```python
from build123d import *

# Parameters (mm, degrees)
BASE_FLANGE1_DEPTH         = 6
SKETCHED_START             = -292.5
SKETCHED_BEND1_OUTLINE_W   = 6
SKETCHED_BEND1_OUTLINE_H   = 180
SKETCHED_BEND1_DEPTH       = 75
SKETCHED_START_2           = 217.5
SKETCHED_BEND1_2_OUTLINE_W = 6
SKETCHED_BEND1_2_OUTLINE_H = 180
SKETCHED_BEND1_2_DEPTH     = 75
SKETCHED_START_3           = -217.5
SKETCHED_BEND1_3_DEPTH     = 6.7366
SKETCHED_START_4           = 210.7634
SKETCHED_BEND1_4_DEPTH     = 6.7366
SKETCHED_START_5           = -91
SKETCHED_BEND1_5_DEPTH     = 182


with BuildPart() as part:
    # Base-Flange1: sheet metal written as solids
    # Sketch1 → Base-Flange1 (new body)
    with BuildSketch(Plane(origin=(0, 0, 0), x_dir=(1, 0, 0), z_dir=(0, 1, 0))):
        with BuildLine():
            Line((-282.5, 90), (282.5, 90))
            ThreePointArc((282.5, 90), (289.571067812, 87.071067812), (292.5, 80))
            Line((292.5, 80), (292.5, -80))
            ThreePointArc((292.5, -80), (289.571067812, -87.071067812), (282.5, -90))
            Line((282.5, -90), (-282.5, -90))
            ThreePointArc((-282.5, -90), (-289.571067812, -87.071067812), (-292.5, -80))
            Line((-292.5, -80), (-292.5, 80))
            ThreePointArc((-292.5, 80), (-289.571067812, 87.071067812), (-282.5, 90))
        make_face()
        with BuildLine():
            Line((-263.3, 55), (-263.3, -55))
            ThreePointArc((-263.3, -55), (-267.5, -59.2), (-271.7, -55))
            Line((-271.7, -55), (-271.7, 55))
            ThreePointArc((-271.7, 55), (-267.5, 59.2), (-263.3, 55))
        make_face(mode=Mode.SUBTRACT)
        with BuildLine():
            Line((-238.3, 55), (-238.3, -55))
            ThreePointArc((-238.3, -55), (-242.5, -59.2), (-246.7, -55))
            Line((-246.7, -55), (-246.7, 55))
            ThreePointArc((-246.7, 55), (-242.5, 59.2), (-238.3, 55))
        make_face(mode=Mode.SUBTRACT)
        with BuildLine():
            Line((246.7, 55), (246.7, -55))
            ThreePointArc((246.7, -55), (242.5, -59.2), (238.3, -55))
            Line((238.3, -55), (238.3, 55))
            ThreePointArc((238.3, 55), (242.5, 59.2), (246.7, 55))
        make_face(mode=Mode.SUBTRACT)
        with BuildLine():
            Line((271.7, 55), (271.7, -55))
            ThreePointArc((271.7, -55), (267.5, -59.2), (263.3, -55))
            Line((263.3, -55), (263.3, 55))
            ThreePointArc((263.3, 55), (267.5, 59.2), (271.7, 55))
        make_face(mode=Mode.SUBTRACT)
        with BuildLine():
            Line((-108.396335225, 50.861970557), (-158.396335225, -59.138029443))
            ThreePointArc((-158.396335225, -59.138029443), (-171.638029443, -64.103664775), (-176.603664775, -50.861970557))
            Line((-176.603664775, -50.861970557), (-126.603664775, 59.138029443))
            ThreePointArc((-126.603664775, 59.138029443), (-113.361970557, 64.103664775), (-108.396335225, 50.861970557))
        make_face(mode=Mode.SUBTRACT)
        with BuildLine():
            Line((-58.396335225, 50.861970557), (-108.396335225, -59.138029443))
            ThreePointArc((-108.396335225, -59.138029443), (-121.638029443, -64.103664775), (-126.603664775, -50.861970557))
            Line((-126.603664775, -50.861970557), (-76.603664775, 59.138029443))
            ThreePointArc((-76.603664775, 59.138029443), (-63.361970557, 64.103664775), (-58.396335225, 50.861970557))
        make_face(mode=Mode.SUBTRACT)
        with BuildLine():
            Line((76.603664775, 59.138029443), (126.603664775, -50.861970557))
            ThreePointArc((126.603664775, -50.861970557), (121.638029443, -64.103664775), (108.396335225, -59.138029443))
            Line((108.396335225, -59.138029443), (58.396335225, 50.861970557))
            ThreePointArc((58.396335225, 50.861970557), (63.361970557, 64.103664775), (76.603664775, 59.138029443))
        make_face(mode=Mode.SUBTRACT)
        with BuildLine():
            Line((126.603664775, 59.138029443), (176.603664775, -50.861970557))
            ThreePointArc((176.603664775, -50.861970557), (171.638029443, -64.103664775), (158.396335225, -59.138029443))
            Line((158.396335225, -59.138029443), (108.396335225, 50.861970557))
            ThreePointArc((108.396335225, 50.861970557), (113.361970557, 64.103664775), (126.603664775, 59.138029443))
        make_face(mode=Mode.SUBTRACT)
    extrude(amount=-BASE_FLANGE1_DEPTH)

    # Sketched Bend1: read off the stored shape, not the designer's step
    # Sketched Bend1 outline → Sketched Bend1 (cut)
    with BuildSketch(Plane.YZ.offset(SKETCHED_START)):
        with Locations((-3, 0)):
            Rectangle(SKETCHED_BEND1_OUTLINE_W, SKETCHED_BEND1_OUTLINE_H)
    extrude(amount=SKETCHED_BEND1_DEPTH, mode=Mode.SUBTRACT)

    # Sketched Bend1 2 outline → Sketched Bend1 2 (cut)
    with BuildSketch(Plane.YZ.offset(SKETCHED_START_2)):
        with Locations((-3, 0)):
            Rectangle(SKETCHED_BEND1_2_OUTLINE_W, SKETCHED_BEND1_2_OUTLINE_H)
    extrude(amount=SKETCHED_BEND1_2_DEPTH, mode=Mode.SUBTRACT)

    # Sketched Bend1 3 outline → Sketched Bend1 3 (add)
    with BuildSketch(Plane.YZ.offset(SKETCHED_START_3)):
        with BuildLine():
            Line((0, 90), (0, -90))
            Line((0, -90), (66.603762445, -90))
            ThreePointArc((66.603762445, -90), (73.674830257, -87.071067812), (76.603762445, -80))
            Line((76.603762445, -80), (76.603762445, 80))
            ThreePointArc((76.603762445, 80), (73.674830257, 87.071067812), (66.603762445, 90))
            Line((66.603762445, 90), (0, 90))
        make_face()
        with BuildLine():
            ThreePointArc((22.403762445, 55), (26.603762445, 59.2), (30.803762445, 55))
            Line((30.803762445, 55), (30.803762445, -55))
            ThreePointArc((30.803762445, -55), (26.603762445, -59.2), (22.403762445, -55))
            Line((22.403762445, -55), (22.403762445, 55))
        make_face(mode=Mode.SUBTRACT)
        with BuildLine():
            ThreePointArc((47.403762445, 55), (51.603762445, 59.2), (55.803762445, 55))
            Line((55.803762445, 55), (55.803762445, -55))
            ThreePointArc((55.803762445, -55), (51.603762445, -59.2), (47.403762445, -55))
            Line((47.403762445, -55), (47.403762445, 55))
        make_face(mode=Mode.SUBTRACT)
    extrude(amount=SKETCHED_BEND1_3_DEPTH)

    # Sketched Bend1 4 outline → Sketched Bend1 4 (add)
    with BuildSketch(Plane.YZ.offset(SKETCHED_START_4)):
        with BuildLine():
            Line((0, 90), (0, -90))
            Line((0, -90), (66.603762445, -90))
            ThreePointArc((66.603762445, -90), (73.674830257, -87.071067812), (76.603762445, -80))
            Line((76.603762445, -80), (76.603762445, 80))
            ThreePointArc((76.603762445, 80), (73.674830257, 87.071067812), (66.603762445, 90))
            Line((66.603762445, 90), (0, 90))
        make_face()
        with BuildLine():
            ThreePointArc((22.403762445, 55), (26.603762445, 59.2), (30.803762445, 55))
            Line((30.803762445, 55), (30.803762445, -55))
            ThreePointArc((30.803762445, -55), (26.603762445, -59.2), (22.403762445, -55))
            Line((22.403762445, -55), (22.403762445, 55))
        make_face(mode=Mode.SUBTRACT)
        with BuildLine():
            ThreePointArc((47.403762445, 55), (51.603762445, 59.2), (55.803762445, 55))
            Line((55.803762445, 55), (55.803762445, -55))
            ThreePointArc((55.803762445, -55), (51.603762445, -59.2), (47.403762445, -55))
            Line((47.403762445, -55), (47.403762445, 55))
        make_face(mode=Mode.SUBTRACT)
    extrude(amount=SKETCHED_BEND1_4_DEPTH)

    # Sketched Bend1 5 outline → Sketched Bend1 5 (cut)
    with BuildSketch(Plane.XY.offset(SKETCHED_START_5)):
        with BuildLine():
            Line((-217.5, -6), (-210.7634, -6))
            ThreePointArc((-210.7634, -6), (-215.526895542, -4.026895542), (-217.5, 0.7366))
            Line((-217.5, 0.7366), (-217.5, -6))
        make_face()
        with BuildLine():
            ThreePointArc((217.5, 0.7366), (215.526895542, -4.026895542), (210.7634, -6))
            Line((210.7634, -6), (217.5, -6))
            Line((217.5, -6), (217.5, 0.7366))
        make_face()
        with BuildLine():
            Line((-210.7634, 0), (-210.7634, 76.603762445))
            Line((-210.7634, 76.603762445), (-211.5, 76.603762445))
            Line((-211.5, 76.603762445), (-211.5, 0.7366))
            ThreePointArc((-211.5, 0.7366), (-211.284254855, 0.215745145), (-210.7634, 0))
        make_face()
        with BuildLine():
            ThreePointArc((210.7634, 0), (211.284254855, 0.215745145), (211.5, 0.7366))
            Line((211.5, 0.7366), (211.5, 76.603762445))
            Line((211.5, 76.603762445), (210.7634, 76.603762445))
            Line((210.7634, 76.603762445), (210.7634, 0))
        make_face()
    extrude(amount=SKETCHED_BEND1_5_DEPTH, mode=Mode.SUBTRACT)


solid = part.part
```
Read the model definition and answer for the solid it produces. Units are mm, in the model's axes. A direction names the side the tool comes from. Coordinates: 2 decimals unless noted, no trailing zeros. Write each loop counter-clockwise with the first axis right and the second up, starting at its lowest first coordinate (ties: lowest second). Pieces come first, ordered by that corner, then holes. Notation, with made-up numbers: (-10.5, 27) -> (6.5, 27) arc R21 cw to (6.5, 31) -> close; hole circle Ø3 at (-18, 22.25). An arc over 180 degrees is marked (long way). Return JSON: item names as keys, results as strings.
1. Determine the mould class of faces 1 (the face through (-214.542, 73.597, -87.148)), 2 (the face through (-217.5, 38, 1)), 3 (the face through (214.458, 73.752, 86.993)), 4 (the face through (-83.046, -2.958, 3.368)) for opening direction Z: pulls with the +Z half, pulls with the -Z half, needs draft (parallel to the pull), parting line crosses it, or undercut.
Found:
{"face 1": "pulls with the -Z half", "face 2": "needs draft", "face 3": "pulls with the +Z half", "face 4": "undercut"}
2. A cutting plane is placed at A-A (y = 26.5). Determine the outline of the cut face in (x, z).
Found:
{"outline": "(-217.5, -90) -> (-211.5, -90) -> (-211.5, -59.2) -> (-217.5, -59.2) -> close; (-217.5, 59.2) -> (-211.5, 59.2) -> (-211.5, 90) -> (-217.5, 90) -> close; (211.5, -90) -> (217.5, -90) -> (217.5, -59.2) -> (211.5, -59.2) -> close; (211.5, 59.2) -> (217.5, 59.2) -> (217.5, 90) -> (211.5, 90) -> close"}
3. A cutting plane is placed at B-B (x = -87). Determine the outline of the cut face in (y, z).
Found:
{"outline": "(-6, -90) -> (0, -90) -> (0, -36.27) -> (-6, -36.27) -> close; (-6, 12.07) -> (0, 12.07) -> (0, 90) -> (-6, 90) -> close"}
4. A cutting plane is placed at D-D (x = 49.5). Determine the outline of the cut face in (y, z), and give its area (3 significant figures).
Found:
{"outline": "(-6, -90) -> (0, -90) -> (0, 90) -> (-6, 90) -> close", "area": "1,080 mm2"}
5. Each of these flat-tipped pins is pushed along its axis until it touches: P1, Ø5, axis at x = 31.5, z = -55.5, coming from the +Y side; P2, Ø5, axis at x = -215, z = 21.5, coming from the -Y side; P3, Ø3, axis at x = 216, z = 2, coming from the -Y side. Where does it stop, or does it pass through?
Found:
{"P1": "y = 0", "P2": "y = -5.77", "P3": "y = -4.87"}
6. Find the intervals of material crossed by line 1 along X through (y, z) = (45, -38.5); line 2 along Y through (x, z) = (-21.5, 47); line 3 along Z through (x, y) = (166.5, -1), in increasing order. Write a range as from..to.
Found:
{"line 1": "-217.5..-211.5, 211.5..217.5", "line 2": "-6..0", "line 3": "-90..28.63, 64.95..90"}
7. A cutting plane is placed at C-C (y = 60). Determine the outline of the cut face in (x, z), and give its area (3 significant figures).
Found:
{"outline": "(-217.5, -90) -> (-211.5, -90) -> (-211.5, 90) -> (-217.5, 90) -> close; (211.5, -90) -> (217.5, -90) -> (217.5, 90) -> (211.5, 90) -> close", "area": "2,160 mm2"}
8. A tool of negligible diameter and unlimited length cuts with its end or side. For faces 5 (the face through (217.5, 38, 1)), 6 (the face through (-211.5, 39, -1)), 7 (the face through (133.746, -2.958, 4.908)), from which of +Z, -Z, +X, -X, +Y, -Y can it reach the whole face along a straight path? Write none if from no direction.
Found:
{"face 5": "+Z, -Z, +X, +Y, -Y", "face 6": "+Z, -Z, +Y", "face 7": "+Y, -Y"}
